Source: CAD feature listing. Evaluate the final solid. Frame: model axes, mm. A direction names the side the tool comes from. Round coordinates to 2 decimals unless told otherwise and drop trailing zeros. Order: outer loops, then holes, each group sorted by start corner. A loop starts at its lowest first (then second) coordinate and runs counter-clockwise, first axis right, second up. Notation, with made-up numbers: (-28.5, -18.75) - (-19.5, -18.75) arc R9 cw to (-19.5, -6.75) - close; hole circle Ø10 at (-20, 56). An arc over 180 degrees is marked (long way). Put each result on its own line as item: value. Start each with the question number.
1) Section A-A on z = 22.5. Output: boundary loops of the cut face in (x, y).
2) Section C-C on z = 0. Output: boundary loops of the cut face in (x, y), then the cut area to 3 significant figures.
3) Line query: probe 1 along X at (y, z) = (-2, -20.5); probe 2 along Z at (x, y) = (7, -6) (3 decimals); probe 3 along X at (y, z) = (-5.25, 0). Output: solid intervals per line, ascending. Write a range as [from, to].
4) Section B-B on x = -24.5. Output: boundary loops of the cut face in (y, z).
5) Contact query for flat-ended pins moving along their axis: P1, Ø3, axis at x = -15.5, z = -33, coming from the -Y side; P2, Ø1, axis at x = -9, z = -2, coming from the +Y side; P3, Ø4, axis at x = -8.5, y = -12, coming from the -Z side; P4, Ø9, axis at x = 33, y = -2.5, coming from the -Z side. Output: stop coordinate, or through.
6) Mould query, pull axis X, two halves, no side actions, for faces 1 (the face through (22.62, -3.94, -27.18)), 2 (the face through (-13.64, -3.94, -0.13)), 3 (the face through (17.6, -3.9, 46.8)). Classes: +X half, -X half, draft (parallel to the pull), parting line (faces both ways), or undercut.
7) Access query for faces 4 (the face through (-22.4, -3.9, -26.8)), 5 (the face through (0.33, -27.86, 7.493)), 6 (the face through (-9.76, -3.94, -2.17)). Directions: +Z, -Z, +X, -X, +Y, -Y. A direction counts if a zero-diameter tool reaches every point of the face in a straight line with its end or side. Return the directions, or none.
8) Section D-D on x = 17. Output: boundary loops of the cut face in (y, z), then the cut area to 3 significant figures.
```python
from build123d import *

# Parameters (mm, degrees)
SKETCH1_R           = 10
BOSS_EXTRUDE1_DEPTH = 8
SKETCH2_R           = 12.5
BOSS_EXTRUDE2_DEPTH = 10
SKETCH3_R           = 7.5
BOSS_EXTRUDE3_DEPTH = 20


with BuildPart() as part:
    # Sketch1 → Boss-Extrude1 (new body)
    with BuildSketch(Plane(origin=(0, 0, 0), x_dir=(1, 0, 0), z_dir=(0, 1, 0))):
        with BuildLine():
            Line((-19.64, -6), (-49.638694584, -6))
            ThreePointArc((-49.638694584, -6), (-49.335912066, -8.122055195), (-48.942454178, -10.229182717))
            ThreePointArc((-48.942454178, -10.229182717), (-34.641016151, -20), (-33.329959182, -37.270817283))
            ThreePointArc((-33.329959182, -37.270817283), (-31.701862163, -38.665125571), (-30.015499715, -39.98837052))
            Line((-30.015499715, -39.98837052), (-15.016152423, -14.00873893))
            ThreePointArc((-15.016152423, -14.00873893), (-6.82, -11.812586508), (-4.623847577, -20.00873893))
            Line((-4.623847577, -20.00873893), (-19.623194869, -45.98837052))
            ThreePointArc((-19.623194869, -45.98837052), (-17.634049903, -46.787180766), (-15.612494996, -47.5))
            ThreePointArc((-15.612494996, -47.5), (0, -40), (15.612494996, -47.5))
            ThreePointArc((15.612494996, -47.5), (17.634049903, -46.787180766), (19.623194869, -45.98837052))
            Line((19.623194869, -45.98837052), (4.623847577, -20.00873893))
            ThreePointArc((4.623847577, -20.00873893), (6.82, -11.812586508), (15.016152423, -14.00873893))
            Line((15.016152423, -14.00873893), (30.015499715, -39.98837052))
            ThreePointArc((30.015499715, -39.98837052), (31.701862163, -38.665125571), (33.329959182, -37.270817283))
            ThreePointArc((33.329959182, -37.270817283), (34.641016151, -20), (48.942454178, -10.229182717))
            ThreePointArc((48.942454178, -10.229182717), (49.335912066, -8.122055195), (49.638694584, -6))
            Line((49.638694584, -6), (19.64, -6))
            ThreePointArc((19.64, -6), (13.64, 0), (19.64, 6))
            Line((19.64, 6), (49.638694584, 6))
            ThreePointArc((49.638694584, 6), (49.335912066, 8.122055195), (48.942454178, 10.229182717))
            ThreePointArc((48.942454178, 10.229182717), (34.641016151, 20), (33.329959182, 37.270817283))
            ThreePointArc((33.329959182, 37.270817283), (31.701862163, 38.665125571), (30.015499715, 39.98837052))
            Line((30.015499715, 39.98837052), (15.016152423, 14.00873893))
            ThreePointArc((15.016152423, 14.00873893), (6.82, 11.812586508), (4.623847577, 20.00873893))
            Line((4.623847577, 20.00873893), (19.623194869, 45.98837052))
            ThreePointArc((19.623194869, 45.98837052), (17.634049903, 46.787180766), (15.612494996, 47.5))
            ThreePointArc((15.612494996, 47.5), (0, 40), (-15.612494996, 47.5))
            ThreePointArc((-15.612494996, 47.5), (-17.634049903, 46.787180766), (-19.623194869, 45.98837052))
            Line((-19.623194869, 45.98837052), (-4.623847577, 20.00873893))
            ThreePointArc((-4.623847577, 20.00873893), (-6.82, 11.812586508), (-15.016152423, 14.00873893))
            Line((-15.016152423, 14.00873893), (-30.015499715, 39.98837052))
            ThreePointArc((-30.015499715, 39.98837052), (-31.701862163, 38.665125571), (-33.329959182, 37.270817283))
            ThreePointArc((-33.329959182, 37.270817283), (-34.641016151, 20), (-48.942454178, 10.229182717))
            ThreePointArc((-48.942454178, 10.229182717), (-49.335912066, 8.122055195), (-49.638694584, 6))
            Line((-49.638694584, 6), (-19.64, 6))
            ThreePointArc((-19.64, 6), (-13.64, 0), (-19.64, -6))
        make_face()
        with Locations(Location((0, 0, 0), (0, 0, 270))):
            Circle(SKETCH1_R, mode=Mode.SUBTRACT)
    extrude(amount=-BOSS_EXTRUDE1_DEPTH)

    # Sketch2 → Boss-Extrude2 (add)
    with BuildSketch(Plane.XZ.offset(8)):
        with Locations(Location((0, 0, 0), (0, 0, 90))):
            Circle(SKETCH2_R)
    extrude(amount=BOSS_EXTRUDE2_DEPTH)

    # Sketch3 → Boss-Extrude3 (add)
    with BuildSketch(Plane.XZ.offset(18)):
        with Locations(Location((0, 0, 0), (0, 0, 270))):
            Circle(SKETCH3_R)
    extrude(amount=BOSS_EXTRUDE3_DEPTH)


solid = part.part
```
Answer sheet:
1. outline: (-33.42, -8) - (-19.92, -8) - (-19.92, 0) - (-33.42, 0) - close; (-6.06, -8) - (6.06, -8) - (6.06, 0) - (-6.06, 0) - close; (19.92, -8) - (33.42, -8) - (33.42, 0) - (19.92, 0) - close
2. outline: (-13.64, -8) - (-12.5, -8) - (-12.5, -18) - (-7.5, -18) - (-7.5, -38) - (7.5, -38) - (7.5, -18) - (12.5, -18) - (12.5, -8) - (13.64, -8) - (13.64, 0) - (10, 0) - (10, -8) - (-10, -8) - (-10, 0) - (-13.64, 0) - close
2. area: 608 mm^2
3. probe 1: [-34.36, -18.76], [-4.91, 4.91], [18.76, 34.36]
3. probe 2: [-41.265, -24.124], [-11.713, -7.141], [7.141, 11.713], [24.124, 41.265]
3. probe 3: [-13.64, -10], [10, 13.64]
4. outline: (-8, -30.44) - (0, -30.44) - (0, -6) - (-8, -6) - close; (-8, 6) - (0, 6) - (0, 30.44) - (-8, 30.44) - close
5. P1: through
5. P2: y = -8
5. P3: z = -10.68
5. P4: z = -39.99
6. face 1: undercut
6. face 2: -X half
6. face 3: +X half
7. face 4: +Y, -Y
7. face 5: -Y
7. face 6: +Y
8. outline: (-8, -47.02) - (0, -47.02) - (0, -41.44) - (-8, -41.44) - close; (-8, -17.44) - (0, -17.44) - (0, -5.39) - (-8, -5.39) - close; (-8, 5.39) - (0, 5.39) - (0, 17.44) - (-8, 17.44) - close; (-8, 41.44) - (0, 41.44) - (0, 47.02) - (-8, 47.02) - close
8. area: 282 mm^2
